Verification items for the finished model (mm, model axes). A direction names the side the tool comes from. Coordinates: 2 decimals unless noted, no trailing zeros. Order: outer loops, then holes, each group sorted by start corner. A loop starts at its lowest first (then second) coordinate and runs counter-clockwise, first axis right, second up. Notation, with made-up numbers: (56.5, -39) -> (96.5, -39) arc R17 ccw to (96.5, -7) -> close; hole circle Ø9 at (-10, 13.5). An arc over 180 degrees is marked (long way). Write item = value, one per line. Start each with the question number.
1. Release check for a two-part mould opening along X. For faces 1 (the flat face through (-9.857, 8, 9)), 2 (the flat face through (-21, 11, 0)), 3 (the flat face through (-14.455, 4, 9)) record: +X half, -X half, draft (parallel to the pull), parting line (faces both ways), or undercut.
2. Cross-section at A-A on y = 4. Record the cut outline in (x, z).
3. Set-up check for faces 4 (the flat face through (-37.315, 4, 9)), 5 (the cylindrical face through (-3.643, 0.884, 8.92)), 6 (the flat face through (-4.8, 1.743, 6.7)), 7 (the flat face through (-46, 1.743, 11)): record each of +Z, -Z, +X, -X, +Y, -Y from which the full face is reachable in a straight line by a thin tool's end or side.
4. Cross-section at B-B on z = 3.5. Record the cut outline in (x, y).
5. Cross-section at C-C on x = -6. Record the cut outline in (y, z), plus the area to 3 significant figures.
6. Go/stop test with flat-tipped pins: P1, Ø4.5, axis at x = -45, z = 4.5, coming from the +Y side; P2, Ø1, axis at x = -20.5, y = 7.5, coming from the -Z side; P3, Ø1.5, axis at y = 12, z = 4.5, coming from the +X side; P4, Ø7, axis at y = 10.5, z = 8.5, coming from the -X side. Record where each tip stops, or that it passes through.
7. Cross-section at D-D on y = 13.75. Record the cut outline in (x, z).
8. Thickness scan on line 1 along X through (y, z) = (3, 14.5); line 2 along X through (y, z) = (1, 4.75); line 3 along Y through (x, z) = (-47, 15.5). Record the ranges inside material, lowest first. Write a range as from..to.
from build123d import *

# Parameters (mm, degrees)
F1_DEPTH = 17.4625
F2_R     = 2.1078217737
F3_DEPTH = 25.4
F4_R     = 2.0502205364
F5_DEPTH = 25.4
F7_DEPTH = 25.4


# Not quite as in the source:
# - a length typed as a fraction of an inch, garbled in the dataset ("3 / 203.2 mm" for 3/8 in), is restored
# - a feature names something its author has since deleted; it is built from what else it names


with BuildPart() as f1:
    # F0 (on Top) → F1 (new body)
    with BuildSketch(Plane.XY):
        Polygon((-14.4545807227, 0), (-1.7545807227, 0), (-1.7545807227, 1.7429942964), (-9.8568759859, 1.7429942964), (-9.8568759859, 15.3656043112), (-41.4793491364, 15.3656043112), (-41.4793491364, 1.7429942964), (-50.0414928719, 1.7429942964), (-50.0145807227, 0), (-37.3145807227, 0), (-37.3145807227, 7.112), (-14.4545807227, 7.112), align=None)
    extrude(amount=F1_DEPTH)

    # F2 (on face) → F3 (cut)
    with BuildSketch(Plane(origin=(0, 1.7429942964, 0), x_dir=(-1, 0, 0), z_dir=(0, 1, 0))):
        with Locations((5.7487357408, 8.8277282193)):
            Circle(F2_R)
    extrude(amount=-F3_DEPTH, mode=Mode.SUBTRACT)

    # F4 (on face) → F5 (cut)
    with BuildSketch(Plane(origin=(0, 1.7429942964, 0), x_dir=(-1, 0, 0), z_dir=(0, 1, 0))):
        with Locations((46.049553901, 7.9207858071)):
            Circle(F4_R)
    extrude(amount=-F5_DEPTH, mode=Mode.SUBTRACT)

    # F6 (on face) → F7 (cut)
    with BuildSketch(Plane(origin=(0, 0, 0), x_dir=(1, 0, 0), z_dir=(0, 0, -1))):
        with BuildLine():
            Line((-15.6063264408, -7.112), (-35.3541379623, -7.112))
            ThreePointArc((-35.3541379623, -7.112), (-25.4802322015, -10.0417717978), (-15.6063264408, -7.112))
        make_face()
    extrude(amount=-F7_DEPTH, mode=Mode.SUBTRACT)


solid = f1.part
Worked out:
q1.face_1 = +X half
q1.face_2 = draft
q1.face_3 = undercut
q2.outline = (-41.48, 0) -> (-37.31, 0) -> (-37.31, 17.46) -> (-41.48, 17.46) -> close; (-14.45, 0) -> (-9.86, 0) -> (-9.86, 17.46) -> (-14.45, 17.46) -> close
q3.face_4 = +Z, -Z, -Y
q3.face_5 = +Y, -Y
q3.face_6 = +Z, -Z, +X, +Y
q3.face_7 = +Z, -Z, -X, +Y
q4.outline = (-50.04, 1.74) -> (-50.01, 0) -> (-37.31, 0) -> (-37.31, 7.11) -> (-35.35, 7.11) arc R18.1 cw to (-15.61, 7.11) -> (-14.45, 7.11) -> (-14.45, 0) -> (-1.75, 0) -> (-1.75, 1.74) -> (-9.86, 1.74) -> (-9.86, 15.37) -> (-41.48, 15.37) -> (-41.48, 1.74) -> close
q5.outline = (0, 0) -> (1.74, 0) -> (1.74, 6.73) -> (0, 6.73) -> close; (0, 10.92) -> (1.74, 10.92) -> (1.74, 17.46) -> (0, 17.46) -> close
q5.area = 23.1 mm²
q6.P1 = 1.74
q6.P2 = through
q6.P3 = -9.86
q6.P4 = -41.48
q7.outline = (-41.48, 0) -> (-9.86, 0) -> (-9.86, 17.46) -> (-41.48, 17.46) -> close
q8.line_1 = -41.48..-37.31, -14.45..-9.86
q8.line_2 = -50.03..-37.31, -14.45..-1.75
q8.line_3 = 0..1.74
